Read the model definition and answer for the solid it produces. Units are mm, in the model's axes. Face numbers are marked on the shaded views. Coordinates: 2 decimals unless noted, no trailing zeros. Write each loop counter-clockwise with the first axis right and the second up, starting at its lowest first coordinate (ties: lowest second). Pieces come first, ordered by that corner, then holes. Notation, with made-up numbers: M 79,51.5 L 84,51.5 A28 cw 84,85.5 Z; hole C -24.75,15.5 d8. An arc over 180 degrees is marked long. Write item = value, one per line.
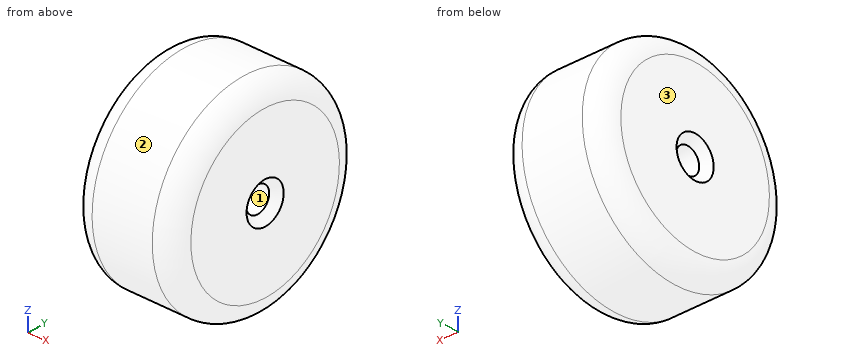
from build123d import *

# Parameters (mm, degrees)
SKETCH1_R           = 40
BOSS_EXTRUDE1_DEPTH = 40
FILLET1_R           = 8
SKETCH2_R           = 5
CUT_EXTRUDE1_DEPTH  = 70.28203236
CHAMFER1_SIZE       = 3


with BuildPart() as part:
    # Sketch1 → Boss-Extrude1 (new body)
    with BuildSketch(Plane(origin=(0, 0, 0), x_dir=(0, 0, -1), z_dir=(1, 0, 0))):
        Circle(SKETCH1_R)
    extrude(amount=BOSS_EXTRUDE1_DEPTH)

    # Fillet1
    fillet1_edges = [part.edges().sort_by_distance(p)[0] for p in [
        (0, 0, 40),
        (40, 0, 40),
    ]]
    fillet(fillet1_edges, radius=FILLET1_R)

    # Sketch2 → Cut-Extrude1 (cut, through all)
    with BuildSketch(Plane(origin=(40, 0, 0), x_dir=(0, 0, -1), z_dir=(1, 0, 0))):
        Circle(SKETCH2_R)
    extrude(amount=-CUT_EXTRUDE1_DEPTH, mode=Mode.SUBTRACT)

    # Chamfer1
    chamfer1_edges = [part.edges().sort_by_distance(p)[0] for p in [
        (0, 0, 5),
        (40, 0, 5),
    ]]
    chamfer(chamfer1_edges, length=CHAMFER1_SIZE)


solid = part.part
Item 1: Find section C-C (x = 31). Determine the outline of the cut face in (y, z).
Worked answers:
outline = C 0,0 d80; hole C 0,0 d10
Item 2: For a pull along Y with two mould halves and no side action, classify the marked faces 1, 2 and 3 as released by +Y, released by -Y, zero draft, split by the parting line, or undercut.
Worked answers:
face_1 = undercut
face_2 = split by the parting line
face_3 = zero draft
Item 3: Flat-ended cylindrical pins translate along their axes: pin 1 (12 mm diameter, centred on x = 36, y = 31.5, fed in from +Z); pin 2 (3 mm diameter, centred on x = 19.5, z = 18.5, fed in from +Y); pin 3 (4 mm diameter, centred on x = 6.5, z = 7, fed in from +Y); pin 4 (5 mm diameter, centred on y = 19.5, z = 28, fed in from -X). Find the tip coordinate at first contact, or state that the pin passes through.
Worked answers:
pin_1 = 30.2
pin_2 = 36.21
pin_3 = 39.64
pin_4 = 0
Item 4: Consider line 1 along Y through (x, z) = (27, 0); line 2 along Z through (x, y) = (21, 4); line 3 along Y through (x, z) = (20, 3.5). Determine where each line is inside the solid, lowest interval first. Write a range as from..to.
Worked answers:
line_1 = -40..-5, 5..40
line_2 = -39.8..-3, 3..39.8
line_3 = -39.85..-3.57, 3.57..39.85
Item 5: Find section A-A (z = 0). Determine the outline of the cut face in (x, y).
Worked answers:
outline = M 0,-32 A8 ccw 8,-40 L 32,-40 A8 ccw 40,-32 L 40,-8 L 37,-5 L 3,-5 L 0,-8 Z; M 0,8 L 3,5 L 37,5 L 40,8 L 40,32 A8 ccw 32,40 L 8,40 A8 ccw 0,32 Z
